Check sheet for the modelled part. Datum: model origin and axes. Units: mm. A direction names the side the tool comes from. Coordinates: 2 decimals unless noted, no trailing zeros. Order: outer loops, then holes, each group sorted by start corner. A loop starts at its lowest first (then second) coordinate and runs counter-clockwise, first axis right, second up.
1. Set-up check for faces 1 (the flat face through (-190, -4, 12.7)), 2 (the flat face through (-486, 47, 12.7)), 3 (the flat face through (130.184, 46.05, 18.961)), 4 (the flat face through (-190, 47, 25.4)), 5 (the flat face through (111.479, 37.814, 6.261)): record each of +Z, -Z, +X, -X, +Y, -Y from which the full face is reachable in a straight line by a thin tool's end or side.
2. Thickness scan on line 1 (Y direction, x = -221, z = 22.75); line 2 (Z direction, x = -511, y = 30); line 3 (X direction, y = 62.5, z = 6.75). Record the ranges inside material, lowest first.
3. Cross-section at B-B (x = 82). Enter the section's corners in (y, z), then the cut area to 3 significant figures.
4. Cross-section at D-D (x = -253). Enter the section's corners in (y, z).
5. Cross-section at A-A (y = 25.5). Enter the section's corners in (x, z), then the cut area to 3 significant figures.
6. Cross-section at C-C (z = 6.25). Enter the section's corners in (x, y).
7. Gauge pin test, flat ends, axial feed: pin 1 Ø4 at (y, z) = (73.5, 22) entering from -X; pin 2 Ø6.5 at (x, z) = (-127, 22) entering from -Y; pin 3 Ø8 at (y, z) = (3.5, 3.5) entering from -X. Record the tip position at first contact, or that the pin passes through.
```python
from build123d import *

# Parameters (mm, degrees)
F1_DEPTH = 12.7
F2_DEPTH = 25.4
F3_DEPTH = 12.7


with BuildPart() as f1:
    # F0 (on Top) → F1 (new body)
    with BuildSketch(Plane.XY):
        Polygon((61.3904680035, 87.9025101712), (-430.82799527, 87.9025101712), (-513.37799527, 5.3525101712), (143.9404680035, 5.3525101712), align=None)
        Polygon((-430.82799527, 87.9025101712), (-457.7687636333, 87.9025101712), (-540.3187636333, 5.3525101712), (-513.37799527, 5.3525101712), align=None)
        Polygon((143.9404680035, 5.3525101712), (-513.37799527, 5.3525101712), (-532.42799527, -13.6974898288), (162.9904680035, -13.6974898288), align=None)
        Polygon((88.3312363667, 87.9025101712), (61.3904680035, 87.9025101712), (143.9404680035, 5.3525101712), (170.8812363667, 5.3525101712), align=None)
    extrude(amount=F1_DEPTH)

    # F0 (on Top) → F2 (join)
    with BuildSketch(Plane.XY):
        Polygon((61.3904680035, 87.9025101712), (-430.82799527, 87.9025101712), (-513.37799527, 5.3525101712), (143.9404680035, 5.3525101712), align=None)
        Polygon((-430.82799527, 87.9025101712), (-457.7687636333, 87.9025101712), (-540.3187636333, 5.3525101712), (-513.37799527, 5.3525101712), align=None)
        Polygon((88.3312363667, 87.9025101712), (61.3904680035, 87.9025101712), (143.9404680035, 5.3525101712), (170.8812363667, 5.3525101712), align=None)
    extrude(amount=F2_DEPTH)

    # F0 (on Top) → F3 (cut)
    with BuildSketch(Plane.XY):
        Polygon((88.3312363667, 87.9025101712), (61.3904680035, 87.9025101712), (143.9404680035, 5.3525101712), (170.8812363667, 5.3525101712), align=None)
        Polygon((-430.82799527, 87.9025101712), (-457.7687636333, 87.9025101712), (-540.3187636333, 5.3525101712), (-513.37799527, 5.3525101712), align=None)
    extrude(amount=F3_DEPTH, mode=Mode.SUBTRACT)


solid = f1.part
```
Data:
1. face 1: +Z, +X, -X, -Y
1. face 2: -Z, -X, +Y
1. face 3: +Z, -Z, +X, +Y
1. face 4: +Z, +X, -X, +Y, -Y
1. face 5: -Z, +X, +Y
2. line 1: y = 5.35 to 87.9
2. line 2: z = 12.7 to 25.4
2. line 3: x = -456.23 to 86.79
3. outline: (-13.7, 0) - (67.29, 0) - (67.29, 12.7) - (87.9, 12.7) - (87.9, 25.4) - (5.35, 25.4) - (5.35, 12.7) - (-13.7, 12.7) - close
3. area: 2,080 mm2
4. outline: (-13.7, 0) - (87.9, 0) - (87.9, 25.4) - (5.35, 25.4) - (5.35, 12.7) - (-13.7, 12.7) - close
5. outline: (-520.17, 12.7) - (-493.23, 12.7) - (-493.23, 0) - (123.79, 0) - (123.79, 12.7) - (150.73, 12.7) - (150.73, 25.4) - (-520.17, 25.4) - close
5. area: 16,400 mm2
6. outline: (-532.43, -13.7) - (162.99, -13.7) - (61.39, 87.9) - (-430.83, 87.9) - close
7. pin 1: stops at x = -474.17
7. pin 2: stops at y = 5.35
7. pin 3: stops at x = -519.23
